Model file for the job. Use its own axes, mm. Give positions to 0.01 mm unless a question says otherwise; leave off trailing zeros. Loops run counter-clockwise (first coordinate to the right, second up) from the corner with the lowest first, then second, coordinate; pieces in that order, holes last. Notation, with made-up numbers: (79, -30.5) - (89, -30.5) arc R20 cw to (89, -8.5) - close; hole circle Ø6 at (38.25, 75). An arc over 180 degrees is marked (long way). Use a Markdown table: item, result.
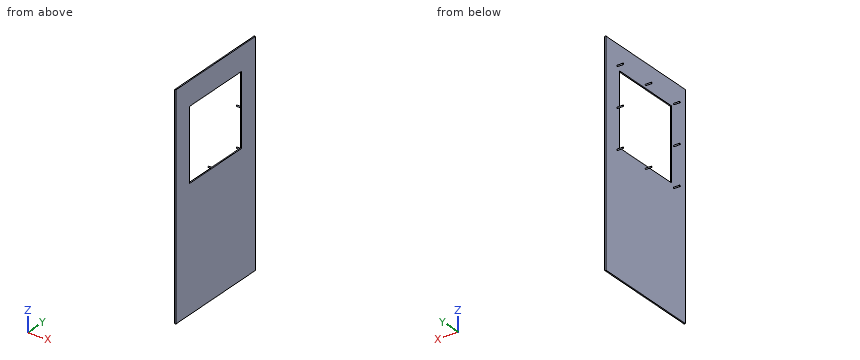
from build123d import *

# Parameters (mm, degrees)
SKETCH1_W           = 547
SKETCH1_H           = 275
BOSS_EXTRUDE1_DEPTH = 3
SKETCH2_W           = 180
SKETCH2_H           = 180
CUT_EXTRUDE1_DEPTH  = 3
SKETCH3_R           = 1.5
BOSS_EXTRUDE2_DEPTH = 15


with BuildPart() as part:
    # Sketch1 → Boss-Extrude1 (new body)
    with BuildSketch(Plane(origin=(0, 0, 0), x_dir=(0, 0, -1), z_dir=(1, 0, 0))):
        Rectangle(SKETCH1_W, SKETCH1_H)
    extrude(amount=BOSS_EXTRUDE1_DEPTH)

    # Sketch2 → Cut-Extrude1 (cut)
    with BuildSketch(Plane(origin=(3, 0, 0), x_dir=(0, 0, -1), z_dir=(1, 0, 0))):
        with Locations((-123.5, 0)):
            Rectangle(SKETCH2_W, SKETCH2_H)
    extrude(amount=-CUT_EXTRUDE1_DEPTH, mode=Mode.SUBTRACT)

    # Sketch3 → Boss-Extrude2 (add)
    with BuildSketch(Plane.ZY):
        with Locations((25.5, 98)):
            Circle(SKETCH3_R)
        with Locations((221.5, -98)):
            Circle(SKETCH3_R)
        with Locations((123.5, 98)):
            Circle(SKETCH3_R)
        with Locations((221.5, 98)):
            Circle(SKETCH3_R)
        with Locations((123.5, -98)):
            Circle(SKETCH3_R)
        with Locations((25.5, -98)):
            Circle(SKETCH3_R)
        with Locations((25.5, 0)):
            Circle(SKETCH3_R)
        with Locations((221.5, 0)):
            Circle(SKETCH3_R)
    extrude(amount=BOSS_EXTRUDE2_DEPTH)


solid = part.part
(1) Slice it at D-D, the plane z = -100. Write the cut outline in (x, y), plus the area to 3 significant figures.
Computed:
| item | result |
|---|---|
| outline | (0, -137.5) - (3, -137.5) - (3, 137.5) - (0, 137.5) - close |
| area | 825 mm² |
(2) Slice it at C-C, the plane x = -6. Write the cut outline in (y, z), plus the area to 3 significant figures.
Computed:
| item | result |
|---|---|
| outline | circle Ø3 at (-98, 25.5); circle Ø3 at (-98, 123.5); circle Ø3 at (-98, 221.5); circle Ø3 at (0, 25.5); circle Ø3 at (0, 221.5); circle Ø3 at (98, 25.5); circle Ø3 at (98, 123.5); circle Ø3 at (98, 221.5) |
| area | 56.5 mm² |
(3) Drill centre lines: probe 1 along X at (y, z) = (-75, -211); probe 2 along Z at (x, y) = (0.5, 39). Where is each one in solid material? Low to high. Write a range as [from, to].
Computed:
| item | result |
|---|---|
| probe 1 | [0, 3] |
| probe 2 | [-273.5, 33.5], [213.5, 273.5] |
(4) Slice it at B-B, the plane y = -60.5. Write the cut outline in (x, z), plus the area to 3 significant figures.
Computed:
| item | result |
|---|---|
| outline | (0, -273.5) - (3, -273.5) - (3, 33.5) - (0, 33.5) - close; (0, 213.5) - (3, 213.5) - (3, 273.5) - (0, 273.5) - close |
| area | 1,100 mm² |
(5) Pin check, flat tips, straight feed: P1, Ø5, axis at y = 32.5, z = -15, coming from the -X side; P2, Ø8, axis at x = -3.5, y = -98, coming from the +Z side; P3, Ø1.5, axis at x = -2, z = -28.5, coming from the +Y side; P4, Ø8, axis at x = -9.5, z = 122, coming from the +Y side. Stop position of each tip, or through.
Computed:
| item | result |
|---|---|
| P1 | x = 0 |
| P2 | z = 273.5 |
| P3 | through |
| P4 | y = 99.5 |
(6) Slice it at A-A, the plane z = 41.5. Write the cut outline in (x, y).
Computed:
| item | result |
|---|---|
| outline | (0, -137.5) - (3, -137.5) - (3, -90) - (0, -90) - close; (0, 90) - (3, 90) - (3, 137.5) - (0, 137.5) - close |
